```python
from build123d import *

# Parameters (mm, degrees)
F1_DEPTH = 34
F2_R     = 1.75
F3_DEPTH = 8.001
F4_SIZE  = 4
F5_SIZE  = 1
F8_R     = 0.6


with BuildPart() as f1:
    # F0 (on Front) → F1 (new body)
    with BuildSketch(Plane.XZ):
        Polygon((0, -5), (0, 0), (-20, 0), (-20, -8), (-15, -8), (-15, -6), (-2.2426406871, -6), (-1.2426406871, -5), align=None)
    extrude(amount=F1_DEPTH)

    # F2 (on face) → F3 (cut, through all)
    with BuildSketch(Plane.XY):
        with Locations((-8, -5)):
            Circle(F2_R)
        with Locations((-8, -27)):
            Circle(F2_R)
    extrude(amount=-F3_DEPTH, mode=Mode.SUBTRACT)

    # F4
    f4_edges = [f1.edges().sort_by_distance(p)[0] for p in [
        (-20, -17, 0),
    ]]
    chamfer(f4_edges, length=F4_SIZE)

    # F5
    f5_edges = [f1.edges().sort_by_distance(p)[0] for p in [
        (-15, -17, -6),
    ]]
    chamfer(f5_edges, length=F5_SIZE)

    # F6: F1 across face


with BuildPart() as f1_1:
    add(f1.part)
    add(f1.part.mirror(Plane(origin=(0, -17, -2.5), x_dir=(0, 1, 0), z_dir=(1, 0, 0))))

    # F8
    f8_edges = [f1_1.edges().sort_by_distance(p)[0] for p in [
        (20, -17, -4),
        (16, -17, 0),
        (-18, 0, -2),
        (-16, -17, 0),
        (-20, -17, -4),
        (-18, -34, -2),
        (-15, 0, -7.5),
        (-14.5, 0, -6.5),
        (-8.12132, 0, -6),
        (-1.742641, 0, -5.5),
        (0, 0, -5),
        (1.742641, 0, -5.5),
        (8.12132, 0, -6),
        (14.5, 0, -6.5),
        (15, 0, -7.5),
        (17.5, 0, -8),
        (20, 0, -6),
        (18, 0, -2),
        (0, 0, 0),
        (-20, 0, -6),
        (-17.5, 0, -8),
        (-17.5, -34, -8),
        (-15, -34, -7.5),
        (-14.5, -34, -6.5),
        (-8.12132, -34, -6),
        (-1.742641, -34, -5.5),
        (0, -34, -5),
        (1.742641, -34, -5.5),
        (8.12132, -34, -6),
        (14.5, -34, -6.5),
        (15, -34, -7.5),
        (17.5, -34, -8),
        (20, -34, -6),
        (18, -34, -2),
        (0, -34, 0),
        (-20, -34, -6),
    ]]
    fillet(f8_edges, radius=F8_R)


solid = f1_1.part
```
Here's how the part is built. I have some questions about the finished solid (model axes, mm). A direction names the side the tool comes from. Give positions to 0.01 mm unless a question says otherwise; leave off trailing zeros. Loops run counter-clockwise (first coordinate to the right, second up) from the corner with the lowest first, then second, coordinate; pieces in that order, holes last. Notation, with made-up numbers: M 44.25,-34.5 L 64.25,-34.5 A28 cw 64.25,-4.5 Z; hole C 44.25,-16.5 d3. An arc over 180 degrees is marked long. Use one line per item in the form item = value. Start each with the question number.
Q1. If we section it at B-B (x = 8): Write out the boundary of the cut face in (y, z).
Q2. Thinking about a two-plate mould opening in X: for faces 1 (the flat face through (-18, -17, -2)), 2 (the flat face through (18, -17, -8)), 3 (the cylindrical face through (-1.774, -0.171, -5.276)), which applies, +X half, -X half, draft (parallel to the pull), parting line (faces both ways), or undercut?
Q3. If we section it at A-A (y = -5): Write out the boundary of the cut face in (x, z).
Q4. Which directions (+Z, -Z, +X, -X, +Y, -Y) give clear straight access to the entire face, cutting with the end or side of a thin tool? Please do faces 4 (the cylindrical face through (14.62, -33.83, -6.36)), 5 (the cylindrical face through (-14.62, -0.17, -6.36)), 6 (the flat face through (-1.75, -16.77, -5.51)).
Q5. If we section it at D-D (x = 4): Write out the boundary of the cut face in (y, z).
Q6. Will these pins go through, and if not, where does the flat tip stop? pin 1 Ø6 at (x, y) = (-8.5, -22) entering from -Z; pin 2 Ø1.2 at (x, y) = (0.5, -11) entering from -Z; pin 3 Ø3 at (x, y) = (8, -27) entering from +Z.
Q7. I need wall thicknesses on line 1 along Y through (x, z) = (8, -4.75); line 2 along X through (y, z) = (-16, -7); line 3 along X through (y, z) = (-25.5, -6.25). Which ranges of each line are inside material? Lowest first, please.
Q8. If we section it at C-C (y = -14): Write out the boundary of the cut face in (x, z), then the cut area to 3 significant figures.
Taken from the geometry:
q1.outline = M -34,-5.4 A0.6 ccw -33.4,-6 L -28.75,-6 L -28.75,0 L -33.4,0 A0.6 ccw -34,-0.6 Z; M -25.25,-6 L -6.75,-6 L -6.75,0 L -25.25,0 Z; M -3.25,-6 L -0.6,-6 A0.6 ccw 0,-5.4 L 0,-0.6 A0.6 ccw -0.6,0 L -3.25,0 Z
q2.face_1 = -X half
q2.face_2 = draft
q2.face_3 = undercut
q3.outline = M -20,-8 L -15,-8 L -15,-7 L -14,-6 L -9.75,-6 L -9.75,0 L -15.75,0 A0.6 ccw -16.18,-0.18 L -19.82,-3.82 A0.6 ccw -20,-4.25 Z; M -6.25,-6 L -2.24,-6 L -1.24,-5 L 1.24,-5 L 2.24,-6 L 6.25,-6 L 6.25,0 L -6.25,0 Z; M 9.75,-6 L 14,-6 L 15,-7 L 15,-8 L 20,-8 L 20,-4.25 A0.6 ccw 19.82,-3.82 L 16.18,-0.18 A0.6 ccw 15.75,0 L 9.75,0 Z
q4.face_4 = -Z, -Y
q4.face_5 = -Z, +Y
q4.face_6 = -Z, +Y, -Y
q5.outline = M -34,-5.4 A0.6 ccw -33.4,-6 L -0.6,-6 A0.6 ccw 0,-5.4 L 0,-0.6 A0.6 ccw -0.6,0 L -33.4,0 A0.6 ccw -34,-0.6 Z
q6.pin_1 = -6
q6.pin_2 = -5
q6.pin_3 = through
q7.line_1 = -34 to -28.75, -25.25 to -6.75, -3.25 to 0
q7.line_2 = -20 to -15, 15 to 20
q7.line_3 = -20 to -14.25, 14.25 to 20
q8.outline = M -20,-8 L -15,-8 L -15,-7 L -14,-6 L -2.24,-6 L -1.24,-5 L 1.24,-5 L 2.24,-6 L 14,-6 L 15,-7 L 15,-8 L 20,-8 L 20,-4.25 A0.6 ccw 19.82,-3.82 L 16.18,-0.18 A0.6 ccw 15.75,0 L -15.75,0 A0.6 ccw -16.18,-0.18 L -19.82,-3.82 A0.6 ccw -20,-4.25 Z
q8.area = 241 mm^2
